Input: part model. Units: mm. Frame: model coordinates. A direction names the side the tool comes from. Coordinates: 2 decimals unless noted, no trailing zeros. Write each loop counter-clockwise with the first axis right and the second up, starting at its lowest first coordinate (ties: lowest second). Pieces come first, ordered by that corner, then holes. Notation, with made-up numbers: (45, -25) - (94, -25) arc R33 ccw to (94, 8) - close; hole circle Ø3 at (47.5, -26.75). An arc over 180 degrees is marked (long way). One line per question, with ' | ' between items. Start each with the question number.
1) Section query A-A on z = -38.1. Return loops of the section in (x, y).
2) Reachability of faces 1 (the cylindrical face through (-32.99, -9.39, 65.34)), 2 (the flat face through (-13, -12.7, 38)) from +Z, -Z, +X, -X, +Y, -Y: full face, straight path, thin tool, end or side. Return the list, or none.
3) Section query D-D on x = 11. Return loops of the section in (y, z), and give its area (3 significant figures).
4) First-contact query: P1, Ø3, axis at y = -7, z = 47.5, coming from the +X side; P2, Ø1.9, axis at y = -15.5, z = 43, coming from the +X side. Flat tips, straight axial feed; report the tip coordinate or a pass-through.
5) Section query C-C on y = -4.5. Return loops of the section in (x, z).
6) Draft query along Z for faces 3 (the flat face through (-1, -19.05, 1)), 4 (the flat face through (0, -9, 76.2)), 5 (the flat face through (-1, -9, -76.2)), 6 (the cylindrical face through (6.827, -6.439, 48.809)). Return one class per face: released by +Z, released by -Z, zero draft, split by the parting line, or undercut.
7) Section query B-B on x = 0. Return loops of the section in (y, z), and give its area (3 significant figures).
8) Line query: line 1 (Z direction, x = 0, y = -5); line 2 (Z direction, x = 0, y = -14.75); line 3 (X direction, y = -8.5, z = -39). Output: solid intervals per line, ascending.
```python
from build123d import *

# Parameters (mm, degrees)
F1_DEPTH = 19.05
F2_R     = 12.7
F3_DEPTH = 19.051
F4_W     = 28.702
F4_H     = 28.702
F4_R     = 12.7
F5_DEPTH = 6.35


with BuildPart() as f1:
    # F0 (on Front) → F1 (new body)
    with BuildSketch(Plane.XZ):
        with BuildLine():
            Line((-44.45, 38.1), (-44.45, -76.2))
            Line((-44.45, -76.2), (44.45, -76.2))
            Line((44.45, -76.2), (44.45, 38.1))
            ThreePointArc((44.45, 38.1), (33.290768, 65.040768), (6.35, 76.2))
            Line((6.35, 76.2), (-6.35, 76.2))
            ThreePointArc((-6.35, 76.2), (-33.290768, 65.040768), (-44.45, 38.1))
        make_face()
    extrude(amount=F1_DEPTH)

    # F2 (on face) → F3 (cut, through all)
    with BuildSketch(Plane.XZ.offset(19.05)):
        with Locations((0, -38.1)):
            Circle(F2_R)
        with Locations((0, 38.1)):
            Circle(F2_R)
    extrude(amount=-F3_DEPTH, mode=Mode.SUBTRACT)

    # F4 (on face) → F5 (cut)
    with BuildSketch(Plane.XZ.offset(19.05)):
        with Locations((0, 38.1)):
            Rectangle(F4_W, F4_H)
        with Locations((0, 38.1)):
            Circle(F4_R, mode=Mode.SUBTRACT)
    extrude(amount=-F5_DEPTH, mode=Mode.SUBTRACT)


solid = f1.part
```
Answer key:
1) outline: (-44.45, -19.05) - (-12.7, -19.05) - (-12.7, 0) - (-44.45, 0) - close; (12.7, -19.05) - (44.45, -19.05) - (44.45, 0) - (12.7, 0) - close
2) face 1: +Z, -X, +Y, -Y | face 2: -Y
3) outline: (-19.05, -76.2) - (0, -76.2) - (0, -44.45) - (-19.05, -44.45) - close; (-19.05, -31.75) - (0, -31.75) - (0, 31.75) - (-12.7, 31.75) - (-12.7, 23.75) - (-19.05, 23.75) - close; (-19.05, 52.45) - (-12.7, 52.45) - (-12.7, 44.45) - (0, 44.45) - (0, 75.92) - (-19.05, 75.92) - close | area: 2,310 mm²
4) P1: x = 43.62 | P2: x = 44.24
5) outline: (-44.45, -76.2) - (44.45, -76.2) - (44.45, 38.1) arc R38.1 ccw to (6.35, 76.2) - (-6.35, 76.2) arc R38.1 ccw to (-44.45, 38.1) - close; hole circle Ø25.4 at (0, -38.1); hole circle Ø25.4 at (0, 38.1)
6) face 3: zero draft | face 4: released by +Z | face 5: released by -Z | face 6: undercut
7) outline: (-19.05, -76.2) - (0, -76.2) - (0, -50.8) - (-19.05, -50.8) - close; (-19.05, -25.4) - (0, -25.4) - (0, 25.4) - (-12.7, 25.4) - (-12.7, 23.75) - (-19.05, 23.75) - close; (-19.05, 52.45) - (-12.7, 52.45) - (-12.7, 50.8) - (0, 50.8) - (0, 76.2) - (-19.05, 76.2) - close | area: 1,910 mm²
8) line 1: -76.2 to -50.8, -25.4 to 25.4, 50.8 to 76.2 | line 2: -76.2 to -50.8, -25.4 to 23.75, 52.45 to 76.2 | line 3: -44.45 to -12.67, 12.67 to 44.45
